from build123d import *

# Parameters (mm, degrees)
SKETCH001_W   = 114
SKETCH001_H   = 5
SKETCH001_W_2 = 5
SKETCH001_H_2 = 104
PAD001_DEPTH  = 90
SKETCH_W      = 114
SKETCH_H      = 5
PAD_DEPTH     = 5
SKETCH002_W   = 114
SKETCH002_H   = 5
PAD002_DEPTH  = 43
SKETCH003_W   = 114
SKETCH003_H   = 5
PAD003_DEPTH  = 43


with BuildPart() as part:
    # Sketch001 → Pad001 (new body)
    with BuildSketch(Plane.XY):
        with Locations((57, 2.5)):
            Rectangle(SKETCH001_W, SKETCH001_H)
        with Locations((2.5, 57)):
            Rectangle(SKETCH001_W_2, SKETCH001_H_2)
        with Locations((111.5, 57)):
            Rectangle(SKETCH001_W_2, SKETCH001_H_2)
        with Locations((57, 111.5)):
            Rectangle(SKETCH001_W, SKETCH001_H)
    extrude(amount=PAD001_DEPTH)

    # Sketch → Pad (new body)
    with BuildSketch(Plane.XY.offset(90)):
        with Locations((57, 111.5)):
            Rectangle(SKETCH_W, SKETCH_H)
        with Locations((57, 2.5)):
            Rectangle(SKETCH_W, SKETCH_H)
    extrude(amount=PAD_DEPTH)

    # Sketch002 → Pad002 (new body)
    with BuildSketch(Plane.XZ):
        with Locations((57, 92.5)):
            Rectangle(SKETCH002_W, SKETCH002_H)
    extrude(amount=PAD002_DEPTH)

    # Sketch003 → Pad003 (new body)
    with BuildSketch(Plane(origin=(0, 114, 0), x_dir=(-1, 0, 0), z_dir=(0, 1, 0))):
        with Locations((-57, 92.5)):
            Rectangle(SKETCH003_W, SKETCH003_H)
    extrude(amount=PAD003_DEPTH)


solid = part.part
Read the model definition and answer for the solid it produces. Units are mm, in the model's axes. A direction names the side the tool comes from. Coordinates: 2 decimals unless noted, no trailing zeros. Write each loop counter-clockwise with the first axis right and the second up, starting at its lowest first coordinate (ties: lowest second). Pieces come first, ordered by that corner, then holes. Notation, with made-up numbers: (-30.5, -32.5) -> (1.5, -32.5) arc R12 cw to (1.5, -20.5) -> close; hole circle Ø5 at (88.25, -24.75). An arc over 180 degrees is marked (long way). Return JSON: item names as keys, results as strings.
(1) The part is cut by section C-C on z = 29. Give the vertices of the cut face in (x, y), then the cut area to 3 significant figures.
Answers below:
{"outline": "(0, 0) -> (114, 0) -> (114, 114) -> (0, 114) -> close; hole (5, 5) -> (109, 5) -> (109, 109) -> (5, 109) -> close", "area": "2,180 mm^2"}
(2) The part is cut by section B-B on x = 90.5. Give the vertices of the cut face in (y, z).
Answers below:
{"outline": "(-43, 90) -> (0, 90) -> (0, 0) -> (5, 0) -> (5, 95) -> (-43, 95) -> close; (109, 0) -> (114, 0) -> (114, 90) -> (157, 90) -> (157, 95) -> (109, 95) -> close"}
(3) The part is cut by section D-D on y = 142. Give the vertices of the cut face in (x, z), then the cut area to 3 significant figures.
Answers below:
{"outline": "(0, 90) -> (114, 90) -> (114, 95) -> (0, 95) -> close", "area": "570 mm^2"}
(4) Which of the six approach directions +Z, -Z, +X, -X, +Y, -Y give full straight-line access (tool end or side, diameter ignored) to faces 4 (the flat face through (56, 114, 44)), 5 (the flat face through (109, 56, 44)), 6 (the flat face through (56, 0, 44))?
Answers below:
{"face 4": "-Z, +X, -X, +Y", "face 5": "+Z, -Z", "face 6": "-Z, +X, -X, -Y"}
(5) Consider line 1 along Y through (x, z) = (49, 27); line 2 along Z through (x, y) = (66.5, 138). Determine where each line is inside the solid, lowest interval first. Write a range as from..to.
Answers below:
{"line 1": "0..5, 109..114", "line 2": "90..95"}
(6) The part is cut by section A-A on y = 90. Give the vertices of the cut face in (x, z).
Answers below:
{"outline": "(0, 0) -> (5, 0) -> (5, 90) -> (0, 90) -> close; (109, 0) -> (114, 0) -> (114, 90) -> (109, 90) -> close"}
(7) Each of these flat-tipped pins is pushed along its axis until it touches: P1, Ø8, axis at x = 97.5, z = 64, coming from the +Y side; P2, Ø5.5, axis at x = 110.5, y = 68.5, coming from the +Z side; P3, Ø10, axis at y = 50, z = 35.5, coming from the -X side. Where does it stop, or does it pass through?
Answers below:
{"P1": "y = 114", "P2": "z = 90", "P3": "x = 0"}
(8) For a pull along X with two mould halves and no side action, classify faces 1 (the flat face through (5, 56, 44)), 2 (the flat face through (0, 56, 47)), 3 (the flat face through (56, -43, 93)) as pulls with the +X half, pulls with the -X half, needs draft (parallel to the pull), parting line crosses it, or undercut.
Answers below:
{"face 1": "undercut", "face 2": "pulls with the -X half", "face 3": "needs draft"}
